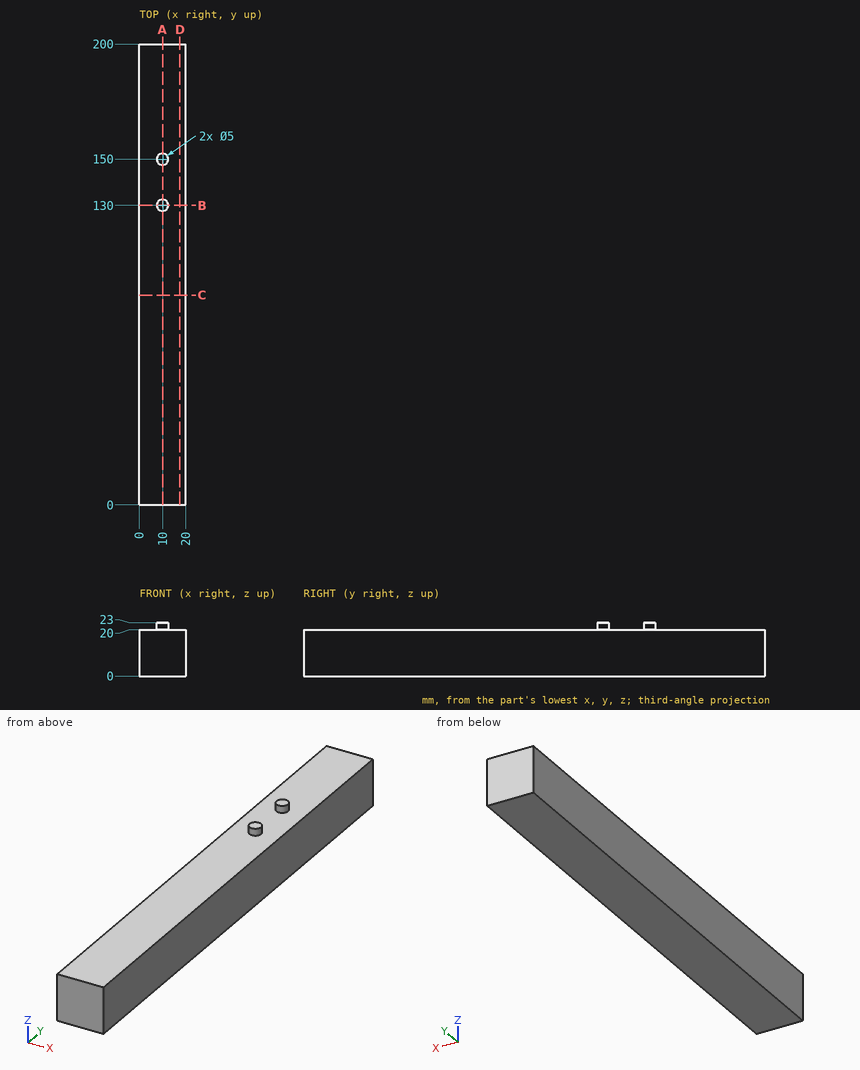
Here's the drawing with two shaded views (mm, measured from the low corner). I have some questions. Coordinates: 2 decimals unless noted, no trailing zeros. Write each loop counter-clockwise with the first axis right and the second up, starting at its lowest first coordinate (ties: lowest second). Pieces come first, ordered by that corner, then holes. Notation, with made-up numbers: M 70,21.25 L 115,21.25 A10 cw 115,39.25 Z; hole C 30,24.25 d11. An arc over 180 degrees is marked long. Write item = value, one per line. Start each with the question number.
Q1. If we section it at A-A, the plane x = 10: Write out the boundary of the cut face in (y, z), then the cut area to 3 significant figures.
Q2. If we section it at B-B, the plane y = 130: Write out the boundary of the cut face in (x, z).
Q3. I'm going to push flat-ended pins straight in: pin 1 (10 mm diameter, centred on y = 114, z = 14, fed in from -X); pin 2 (10 mm diameter, centred on x = 14, y = 118.5, fed in from +Z). Where does each tip first touch, or does it pass through?
Q4. If I drill on L1, parallel to Z at x = 3, y = 64; L2, parallel to Y at x = 12.25, z = 22.25, over which ranges is the centre line in solid material (lowest first)? Write a range as [from, to].
Q5. If we section it at C-C, the plane y = 91: Write out the boundary of the cut face in (x, z), then the cut area to 3 significant figures.
Q6. If we section it at D-D, the plane x = 17.5: Write out the boundary of the cut face in (y, z).
Check sheet entries:
q1.outline = M 0,0 L 200,0 L 200,20 L 152.5,20 L 152.5,23 L 147.5,23 L 147.5,20 L 132.5,20 L 132.5,23 L 127.5,23 L 127.5,20 L 0,20 Z
q1.area = 4,030 mm²
q2.outline = M 0,0 L 20,0 L 20,20 L 12.5,20 L 12.5,23 L 7.5,23 L 7.5,20 L 0,20 Z
q3.pin_1 = 0
q3.pin_2 = 20
q4.L1 = [0, 20]
q4.L2 = [128.91, 131.09], [148.91, 151.09]
q5.outline = M 0,0 L 20,0 L 20,20 L 0,20 Z
q5.area = 400 mm²
q6.outline = M 0,0 L 200,0 L 200,20 L 0,20 Z
